```python
from build123d import *

# Parameters (mm, degrees)
SKETCH2_R           = 1
SKETCH2_R_2         = 2
BOSS_EXTRUDE1_DEPTH = 5


with BuildPart() as part:
    # Sketch2 → Boss-Extrude1 (new, symmetric)
    with BuildSketch(Plane.XY):
        Polygon((-17.5, 8.5), (-19.5, 6.5), (-19.5, -6.5), (-17.5, -8.5), (17.5, -8.5), (19.5, -6.5), (19.5, 6.5), (17.5, 8.5), align=None)
        Circle(SKETCH2_R, mode=Mode.SUBTRACT)
        with Locations((-13.5, -5.5)):
            Circle(SKETCH2_R, mode=Mode.SUBTRACT)
        with Locations((-15.5, 6.5)):
            Circle(SKETCH2_R, mode=Mode.SUBTRACT)
        with Locations((-9.5, 3.5)):
            Circle(SKETCH2_R_2, mode=Mode.SUBTRACT)
        with Locations((7.5, -2.5)):
            Circle(SKETCH2_R_2, mode=Mode.SUBTRACT)
        with Locations((15.5, -4.5)):
            Circle(SKETCH2_R, mode=Mode.SUBTRACT)
        with Locations((11.5, 3.5)):
            Circle(SKETCH2_R, mode=Mode.SUBTRACT)
    extrude(amount=BOSS_EXTRUDE1_DEPTH, both=True)


solid = part.part
```
The model under review builds one solid part; all positions refer to its coordinate system, in mm. Give positions to 0.01 mm unless a question says otherwise; leave off trailing zeros. Write each loop counter-clockwise with the first axis right and the second up, starting at its lowest first coordinate (ties: lowest second). Pieces come first, ordered by that corner, then holes. Notation, with made-up numbers: M 73,-26 L 109,-26 A17 ccw 109,-18 Z; hole C 12.5,-25 d9. An arc over 180 degrees is marked long. Write each question's results on one line, items separated by ' | '. Start each with the question number.
1. Mouldability with a two-part tool opening along X and no side actions: class faces 1 (the flat face through (-18, 8, 0)), 2 (the flat face through (0, -8.5, 0)), 3 (the cylindrical face through (16.454, -4.2, -0.07)), 4 (the cylindrical face through (10.5, 3.5, -0.1)) as released by +X, released by -X, zero draft, split by the parting line, or undercut.
2. We need section C-C (z = 0.75). Write out the cut boundary in (x, y), and give its area (3 significant figures).
3. We need section B-B (x = 7.5). Write out the cut boundary in (y, z).
4. For probe 1 along Y at (x, z) = (11.5, -1.75); probe 2 along Y at (x, z) = (0, 1.25); probe 3 along X at (y, z) = (-0.25, -4.5), list the stretches that pass through material, from the lowest coordinate up. Write a range as [from, to].
5. We need section D-D (y = -7.25). Write out the cut boundary in (x, z).
6. We need section A-A (y = 0). Write out the cut boundary in (x, z), and give its area (3 significant figures).
Results found:
1) face 1: released by -X | face 2: zero draft | face 3: undercut | face 4: undercut
2) outline: M -19.5,-6.5 L -17.5,-8.5 L 17.5,-8.5 L 19.5,-6.5 L 19.5,6.5 L 17.5,8.5 L -17.5,8.5 L -19.5,6.5 Z; hole C -15.5,6.5 d2; hole C -13.5,-5.5 d2; hole C -9.5,3.5 d4; hole C 0,0 d2; hole C 7.5,-2.5 d4; hole C 11.5,3.5 d2; hole C 15.5,-4.5 d2 | area: 614 mm^2
3) outline: M -8.5,-5 L -4.5,-5 L -4.5,5 L -8.5,5 Z; M -0.5,-5 L 8.5,-5 L 8.5,5 L -0.5,5 Z
4) probe 1: y = [-8.5, 2.5], [4.5, 8.5] | probe 2: y = [-8.5, -1], [1, 8.5] | probe 3: x = [-19.5, -0.97], [0.97, 19.5]
5) outline: M -18.75,-5 L 18.75,-5 L 18.75,5 L -18.75,5 Z
6) outline: M -19.5,-5 L -1,-5 L -1,5 L -19.5,5 Z; M 1,-5 L 19.5,-5 L 19.5,5 L 1,5 Z | area: 370 mm^2
